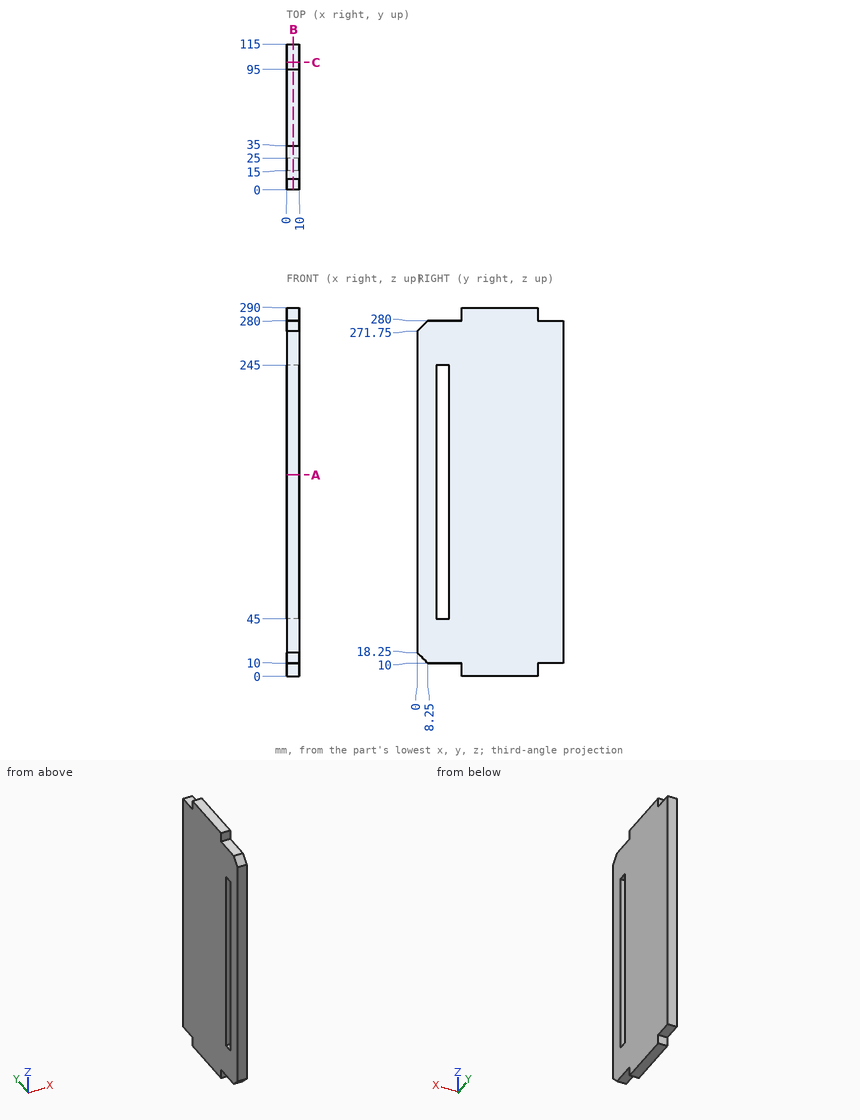
Answer from the drawing. Dimensions are ordinates in mm from the lowest x, y and z of the part. Give positions to 0.01 mm unless a question says otherwise; leave off trailing zeros. Order: outer loops, then holes, each group sorted by start corner. A loop starts at its lowest first (then second) coordinate and runs counter-clockwise, first axis right, second up.
(1) Straight lines are drawn through the part: L1, parallel to Y at x = 8.5, z = 219.5; L2, parallel to Z at x = 6.25, y = 21; L3, parallel to Z at x = 3.5, y = 27. For each, find the intervals that lie inside material, in ascending order.
(2) Find section C-C (y = 100.5). Give the vertices of the cut face in (x, z), plus the area to 3 significant figures.
(3) Find section B-B (x = 5.25). Give the vertices of the cut face in (y, z).
(4) Given pin 1 (1.5 mm diameter, centred on y = 93.5, z = 199, fed in from -X); pin 2 (3 mm diameter, centred on x = 6.5, y = 20.5, fed in from -Z); pin 3 (3 mm diameter, centred on x = 5.5, z = 287, fed in from +Y); pin 4 (3 mm diameter, centred on x = 4, z = 286.5, fed in from -Y), each flat-ended and moving along its own axis, determine where each tip first touches the part or whether it passes through.
(5) Find section A-A (z = 158.5). Give the vertices of the cut face in (x, y).
Result sheet:
1. L1: y = 0 to 15, 25 to 115
1. L2: z = 10 to 45, 245 to 280
1. L3: z = 10 to 280
2. outline: (0, 10) - (10, 10) - (10, 280) - (0, 280) - close
2. area: 2,700 mm2
3. outline: (0, 18.25) - (8.25, 10) - (35, 10) - (35, 0) - (95, 0) - (95, 10) - (115, 10) - (115, 280) - (95, 280) - (95, 290) - (35, 290) - (35, 280) - (8.25, 280) - (0, 271.75) - close; hole (15, 45) - (25, 45) - (25, 245) - (15, 245) - close
4. pin 1: stops at x = 0
4. pin 2: stops at z = 10
4. pin 3: stops at y = 95
4. pin 4: stops at y = 35
5. outline: (0, 0) - (10, 0) - (10, 15) - (0, 15) - close; (0, 25) - (10, 25) - (10, 115) - (0, 115) - close
